Read the model definition and answer for the solid it produces. Units are mm, in the model's axes. A direction names the side the tool comes from. Give positions to 0.01 mm unless a question says otherwise; leave off trailing zeros. Order: outer loops, then holes, each group sorted by start corner. A loop starts at its lowest first (then second) coordinate and runs counter-clockwise, first axis right, second up. Notation, with made-up numbers: M 13,-26.75 L 24,-26.75 A9 ccw 24,-16.75 Z; hole C -33,59 d7. An arc over 180 degrees is marked long. One line per item, written item: value. Start each with the question number.
from build123d import *

# Parameters (mm, degrees)
F0_W     = 35
F0_H     = 35
F1_DEPTH = 7
F2_W     = 5
F2_H     = 5
F3_DEPTH = 5
F4_R     = 15
F5_DEPTH = 5.7
F6_R     = 1.5
F7_DEPTH = 25
F8_W     = 20
F8_H     = 5
F9_DEPTH = 10
F10_R    = 2


with BuildPart() as f1:
    # F0 (on Top) → F1 (new body)
    with BuildSketch(Plane.XY):
        with Locations((-9.063598, -1.130828)):
            Rectangle(F0_W, F0_H)
    extrude(amount=F1_DEPTH)

    # F2 (on face) → F3 (cut)
    with BuildSketch(Plane.XY.offset(7)):
        with Locations((-24.063598, -16.130828)):
            Rectangle(F2_W, F2_H)
        with Locations((5.936402, 13.869172)):
            Rectangle(F2_W, F2_H)
    extrude(amount=-F3_DEPTH, mode=Mode.SUBTRACT)

    # F4 (on face) → F5 (cut)
    with BuildSketch(Plane.XY.offset(7)):
        with Locations((-9.063598, -1.130828)):
            Circle(F4_R)
    extrude(amount=-F5_DEPTH, mode=Mode.SUBTRACT)

    # F6 (on face) → F7 (cut)
    with BuildSketch(Plane.XY.offset(2)):
        with Locations((-24.063598, -16.130828)):
            Circle(F6_R)
        with Locations((5.936402, 13.869172)):
            Circle(F6_R)
    extrude(amount=-F7_DEPTH, mode=Mode.SUBTRACT)

    # F8 (on face) → F9 (cut)
    with BuildSketch(Plane.XZ.offset(18.630828)):
        with Locations((-10.563598, 3.8)):
            Rectangle(F8_W, F8_H)
    extrude(amount=-F9_DEPTH, mode=Mode.SUBTRACT)

    # F10
    f10_edges = [f1.edges().sort_by_distance(p)[0] for p in [
        (8.436402, -18.630828, 3.5),
        (-26.563598, -18.630828, 1),
        (8.436402, 16.369172, 1),
        (-26.563598, 16.369172, 3.5),
    ]]
    fillet(f10_edges, radius=F10_R)


solid = f1.part
Q1. Find section A-A, the plane x = -11. Give the vertices of the cut face in (y, z), then the cut area to 3 significant figures.
Q2. Each of these flat-tipped pins is pushed along its axis until it touches: pin 1 (2.5 mm diameter, centred on x = 6, y = 14.5, fed in from +Z); pin 2 (1.8 mm diameter, centred on x = 5.94, y = 13.87, fed in from -Z); pin 3 (2.5 mm diameter, centred on y = 13.5, z = 3.5, fed in from +X); pin 4 (1.5 mm diameter, centred on y = -17, z = 5, fed in from -X). Where does it stop, or does it pass through?
Q3. Consider probe 1 along Z at (x, y) = (-18, -15); probe 2 along Z at (x, y) = (-0.5, 5); probe 3 along X at (y, z) = (-12.5, 6.25). Determine where each line is inside the solid, lowest interval first.
Q4. A tool of negligible diameter and unlimited length cuts with its end or side. For faces 5 (the flat face through (-13, -16, 6.3)), 6 (the flat face through (3.436, 14, 5)), 7 (the flat face through (-24, -13.631, 5)), 8 (the flat face through (-6, -18.631, 1)), 9 (the cylindrical face through (-25.99, 15.77, 3.55)), from which of +Z, -Z, +X, -X, +Y, -Y can it reach the whole face along a straight path? Write none if from no direction.
Q5. Find section C-C, the plane y = 1. Give the vertices of the cut face in (x, z), then the cut area to 3 significant figures.
Q6. Find section B-B, the plane z = 4.5. Give the vertices of the cut face in (x, y).
Q7. Determine the mould class of faces 1 (the flat face through (-26.564, -1, 3)), 2 (the cylindrical face through (-11.02, 13.74, 4.19)), 3 (the flat face through (6, 12, 2)), 4 (the flat face through (-9, -3, 1.3)) for opening direction X: released by +X, released by -X, zero draft, split by the parting line, or undercut.
Q8. Find section D-D, the plane x = -18. Give the vertices of the cut face in (y, z), then the cut area to 3 significant figures.
Evaluation:
1. outline: M -18.63,0 L 16.37,0 L 16.37,7 L 13.74,7 L 13.74,1.3 L -18.63,1.3 Z; M -18.63,6.3 L -16.01,6.3 L -16.01,7 L -18.63,7 Z
1. area: 62.3 mm2
2. pin 1: z = 2
2. pin 2: through
2. pin 3: x = 3.44
2. pin 4: x = -21.56
3. probe 1: 0 to 1.3, 6.3 to 7
3. probe 2: 0 to 1.3
3. probe 3: -26.56 to -20.56, 0.72 to 8.44
4. face 5: -Y
4. face 6: +Z, +X, +Y
4. face 7: +Z, -X, -Y
4. face 8: +Z, -Z, +X, -X, -Y
4. face 9: +Z, -Z, -X, +Y
5. outline: M -26.56,0 L 8.44,0 L 8.44,7 L 5.78,7 L 5.78,1.3 L -23.91,1.3 L -23.91,7 L -26.56,7 Z
5. area: 75.7 mm2
6. outline: M -26.56,-13.63 L -21.56,-13.63 L -21.56,-18.63 L -20.56,-18.63 L -20.56,-10.76 A15 cw long -0.56,-13.49 L -0.56,-18.63 L 6.44,-18.63 A2 ccw 8.44,-16.63 L 8.44,11.37 L 3.44,11.37 L 3.44,16.37 L -24.56,16.37 A2 ccw -26.56,14.37 Z
7. face 1: released by -X
7. face 2: undercut
7. face 3: zero draft
7. face 4: undercut
8. outline: M -18.63,0 L 16.37,0 L 16.37,7 L 10.92,7 L 10.92,1.3 L -18.63,1.3 Z; M -18.63,6.3 L -13.18,6.3 L -13.18,7 L -18.63,7 Z
8. area: 80.4 mm2
